```python
from build123d import *

# Parameters (mm, degrees)
SKETCH_2_R          = 3
EXTRUDE_1_DEPTH     = 6
SKETCH_3_R          = 5
EXTRUDE_2_DEPTH     = 29.58
SKETCH_4_R          = 2.55
CUT_EXTRUDE_1_DEPTH = 55.029865815


with BuildPart() as part:
    # 草图2 → 凸台-拉伸1 (new body)
    with BuildSketch(Plane.XY):
        with BuildLine():
            Line((26.49133381, -23.443703305), (-3.03527618, -15.532072003))
            ThreePointArc((-3.03527618, -15.532072003), (-5.173413361, -14.103414414), (-6, -11.668368698))
            Line((-6, -11.668368698), (-6, 2))
            ThreePointArc((-6, 2), (-4.828427125, 4.828427125), (-2, 6))
            Line((-2, 6), (39.5, 6))
            Line((39.5, 6), (39.5, -23.58))
            Line((39.5, -23.58), (27.52660999, -23.58))
            ThreePointArc((27.52660999, -23.58), (27.004505221, -23.545779445), (26.49133381, -23.443703305))
        make_face()
        Circle(SKETCH_2_R, mode=Mode.SUBTRACT)
        with Locations((20, 0)):
            Circle(SKETCH_2_R, mode=Mode.SUBTRACT)
        with Locations((20, -12.5)):
            Circle(SKETCH_2_R, mode=Mode.SUBTRACT)
    extrude(amount=EXTRUDE_1_DEPTH)

    # 草图3 → 凸台-拉伸2 (add, through all)
    with BuildSketch(Plane(origin=(0, 6, 0), x_dir=(1, 0, 0), z_dir=(0, 1, 0))):
        with Locations((39.5, -3)):
            Circle(SKETCH_3_R)
    extrude(amount=-EXTRUDE_2_DEPTH)

    # 草图4 → 切除-拉伸1 (cut, through all)
    with BuildSketch(Plane(origin=(0, 6, 0), x_dir=(1, 0, 0), z_dir=(0, 1, 0))):
        with Locations(Location((39.5, -3, 0), (0, 0, 270))):
            Circle(SKETCH_4_R)
    extrude(amount=-CUT_EXTRUDE_1_DEPTH, mode=Mode.SUBTRACT)


solid = part.part
```
Geometry check sheet. Reference: the model listing, model coordinates, mm. A direction names the side the tool comes from. Coordinates: 2 decimals unless noted, no trailing zeros. Order: outer loops, then holes, each group sorted by start corner. A loop starts at its lowest first (then second) coordinate and runs counter-clockwise, first axis right, second up. Notation, with made-up numbers: (81, -31) - (95, -31) arc R10 ccw to (95, -18) - close; hole circle Ø4 at (81.25, 37.25). An arc over 180 degrees is marked (long way). Answer in a Markdown table with one row per item. Add a question column.
1. Section check D-D (x = 20). Enter the section's corners in (y, z).
2. Material ranges on L1, parallel to X at y = -12.75, z = 3; L2, parallel to X at y = -14, z = 2; L3, parallel to Y at x = 18.5, z = 4, recorded low to high. Write a range as [from, to].
3. Draft check along X on faces 1 (the face through (15, -9, 6)), 2 (the face through (17, -12.4, 3)), 3 (the face through (-5.151, -14.132, 2.958)). Enter one of: +X half, -X half, draft (parallel to the pull), parting line (faces both ways), or undercut.
4. Section check A-A (z = 3). Enter the section's corners in (x, y).
5. Gauge pin test, flat ends, axial feed: pin 1 Ø1 at (y, z) = (-12.5, 3) entering from -X; pin 2 Ø3 at (x, y) = (25.5, -17) entering from +Z; pin 3 Ø8 at (x, y) = (0, 0) entering from -Z. Record the tip position at first contact, or that the pin passes through.
6. Access from +Z, -Z, +X, -X, +Y, -Y to the whole of each face (thin tool, end or side, straight path). Record for faces 4 (the face through (17, 0, 3)), 5 (the face through (15, -9, 0)).
7. Section check C-C (y = -13.5). Enter the section's corners in (x, z).
8. Section check B-B (x = 39.5). Enter the section's corners in (y, z), plus the area to 3 significant figures.
Data:
| question | item | result |
|---|---|---|
| 1 | outline | (-21.7, 0) - (-15.5, 0) - (-15.5, 6) - (-21.7, 6) - close; (-9.5, 0) - (-3, 0) - (-3, 6) - (-9.5, 6) - close; (3, 0) - (6, 0) - (6, 6) - (3, 6) - close |
| 2 | L1 | x = [-5.85, 17.01], [22.99, 36.95], [42.05, 44.5] |
| 2 | L2 | x = [-5.25, 17.4], [22.6, 37.15], [41.85, 44.4] |
| 2 | L3 | y = [-21.3, -15.1], [-9.9, -2.6], [2.6, 6] |
| 3 | face 1 | draft |
| 3 | face 2 | undercut |
| 3 | face 3 | -X half |
| 4 | outline | (-6, -11.67) arc R4 ccw to (-3.04, -15.53) - (26.49, -23.44) arc R4 ccw to (27.53, -23.58) - (36.95, -23.58) - (36.95, 6) - (-2, 6) arc R4 ccw to (-6, 2) - close; (42.05, -23.58) - (44.5, -23.58) - (44.5, 6) - (42.05, 6) - close; hole circle Ø6 at (0, 0); hole circle Ø6 at (20, -12.5); hole circle Ø6 at (20, 0) |
| 5 | pin 1 | stops at x = -5.99 |
| 5 | pin 2 | stops at z = 6 |
| 5 | pin 3 | stops at z = 0 |
| 6 | face 4 | +Z, -Z |
| 6 | face 5 | -Z, -X, +Y, -Y |
| 7 | outline | (-5.56, 0) - (17.17, 0) - (17.17, 6) - (-5.56, 6) - close; (22.83, 0) - (35.5, 0) arc R5 ccw (long way) to (35.5, 6) - (22.83, 6) - close; hole circle Ø5.1 at (39.5, 3) |
| 8 | outline | (-23.58, -2) - (6, -2) - (6, 0.45) - (-23.58, 0.45) - close; (-23.58, 5.55) - (6, 5.55) - (6, 8) - (-23.58, 8) - close |
| 8 | area | 145 mm² |
